Could you check a few things on this model? Use its own coordinates, in mm. Face numbers are marked on the shaded views. A direction names the side the tool comes from. Round coordinates to 2 decimals unless told otherwise and drop trailing zeros. One line per item, written item: value.
from build123d import *

# Parameters (mm, degrees)
SKETCH_1_W           = 50
SKETCH_1_H           = 35
EXTRUDE_1_DEPTH      = 51.03
SKETCH_2_W           = 10
SKETCH_2_H           = 5
CUT_EXTRUDE_1_DEPTH  = 51.03
CUT_EXTRUDE_16_DEPTH = 60.458480472
CUT_EXTRUDE_17_DEPTH = 67.738751278
SKETCH_13_W          = 41.03
SKETCH_13_H          = 5
CUT_EXTRUDE_18_DEPTH = 10
SKETCH_14_R          = 1
CUT_EXTRUDE_19_DEPTH = 56.22690393


with BuildPart() as part:
    # 草图1 → 凸台-拉伸1 (new body)
    with BuildSketch(Plane.XY):
        Rectangle(SKETCH_1_W, SKETCH_1_H)
    extrude(amount=EXTRUDE_1_DEPTH)

    # 草图2 → 切除-拉伸1 (cut)
    with BuildSketch(Plane(origin=(0, 17.5, 0), x_dir=(1, 0, 0), z_dir=(0, 1, 0))):
        with Locations((20, -2.5)):
            Rectangle(SKETCH_2_W, SKETCH_2_H)
        with Locations((20, -48.53)):
            Rectangle(SKETCH_2_W, SKETCH_2_H)
    extrude(amount=-CUT_EXTRUDE_1_DEPTH, mode=Mode.SUBTRACT)

    # 草图3 → 切除-拉伸16 (cut, through all)
    with BuildSketch(Plane.XY.offset(51.03)):
        with BuildLine():
            add(Edge.make_bspline(
                [(15, 17.5), (-24.901617215, 9.03072155), (-25, -17.5)],
                knots=[0, 0, 0, 0.995080861, 0.995080861, 0.995080861], degree=2))
            Line((15, 17.5), (-25, 17.5))
            Line((-25, 17.5), (-25, -17.5))
        make_face()
    extrude(amount=-CUT_EXTRUDE_16_DEPTH, mode=Mode.SUBTRACT)

    # 草图11 → 切除-拉伸17 (cut, through all)
    with BuildSketch(Plane.XZ.offset(17.5)):
        Polygon((-25, 35.515), (15, 51.03), (-25, 51.03), align=None)
        Polygon((-25, 0), (15, 0), (-25, 15.515), align=None)
    extrude(amount=-CUT_EXTRUDE_17_DEPTH, mode=Mode.SUBTRACT)

    # 草图13 → 切除-拉伸18 (cut)
    with BuildSketch(Plane(origin=(25, 0, 0), x_dir=(0, 0, -1), z_dir=(1, 0, 0))):
        with Locations((-25.515, 15)):
            Rectangle(SKETCH_13_W, SKETCH_13_H)
    extrude(amount=-CUT_EXTRUDE_18_DEPTH, mode=Mode.SUBTRACT)

    # 草图14 → 切除-拉伸19 (cut, through all)
    with BuildSketch(Plane.XY.offset(46.03)):
        with Locations((23, 10.5)):
            Circle(SKETCH_14_R)
        with Locations((23, -15.5)):
            Circle(SKETCH_14_R)
    extrude(amount=-CUT_EXTRUDE_19_DEPTH, mode=Mode.SUBTRACT)


solid = part.part
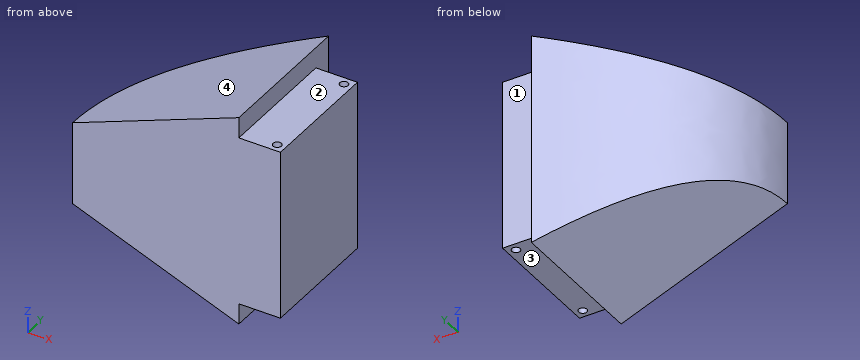
(1) For the marked faces 1, 2, 3 and 4, which set-ups out of +Z, -Z, +X, -X, +Y, -Y let a thin tool reach every point of the face, with its end or its side?
Recorded:
face 1: +Z, -Z, +X, +Y
face 2: +Z, +X, +Y, -Y
face 3: -Z, +X, +Y, -Y
face 4: +Z, -X, +Y, -Y
(2) If we section it at A-A, the plane z = 39: Give the number of separate pieces and of enclosed holes in the cut face, then the cut area to 3 significant figures.
Recorded:
separate pieces: 1
enclosed holes: 2
area: 1,210 mm²
(3) I'm going to push flat-ended pins straight in: pin 1 Ø8 at (y, z) = (13.5, 43) entering from -X; pin 2 Ø2.5 at (x, y) = (23, -15.5) entering from +Z; pin 3 Ø5 at (x, y) = (14, 7) entering from -Z. Where does each tip first touch, or does it pass through?
Recorded:
pin 1: x = -7.67
pin 2: z = 46.03
pin 3: z = 0
(4) If I drill on L1, parallel to Y at x = 23, z = 15; L2, parallel to Z at x = 15.5, y = 2.5; L3, parallel to X at y = 10, z = 31, over which ranges is the centre line in solid material (lowest first)?
Recorded:
L1: -17.5 to -16.5, -14.5 to 9.5, 11.5 to 12.5
L2: 5 to 46.03
L3: -6.9 to 22.13, 23.87 to 25
